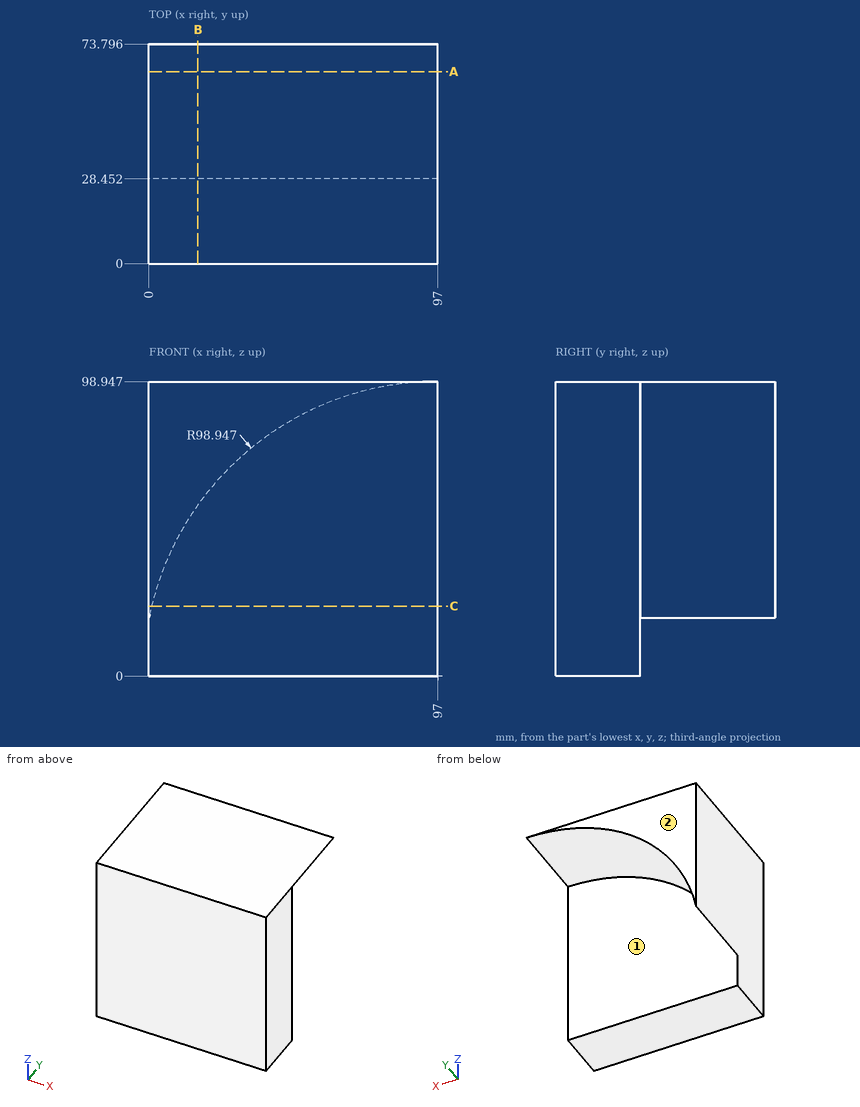
Source: three-view drawing plus pictorial views. Frame: mm from the lowest corner of the part. A direction names the side the tool comes from. Round coordinates to 2 decimals unless told otherwise and drop trailing zeros. Loops run counter-clockwise (first coordinate to the right, second up) from the corner with the lowest first, then second, coordinate; pieces in that order, holes last. Notation, with made-up numbers: M 47.25,45.25 L 100.25,45.25 A15 cw 100.25,52.25 Z; hole C 61.5,51 d8. An arc over 180 degrees is marked long. Answer as CSV lines item,"result". Start each with the question number.
(1) First-contact query: pin 1 (2 mm diameter, centred on x = 49, z = 72.5, fed in from +Y); pin 2 (12 mm diameter, centred on x = 26.5, y = 36, fed in from -Z) (1 decimal); pin 3 (1 mm diameter, centred on x = 51, y = 60.5, fed in from -Z). Flat tips, straight axial feed; report the tip coordinate or a pass-through.
(2) Reachability of the marked faces 1 and 2 from +Z, -Z, +X, -X, +Y, -Y: full face, straight path, thin tool, end or side. Return the list, or none.
(3) Section C-C, the plane z = 23.5. Output: boundary loops of the cut face in (x, y).
(4) Line query: line 1 (Y direction, x = 52.5, z = 86); line 2 (Z direction, x = 53, y = 58) (1 decimal); line 3 (Z direction, x = 9, y = 53). Output: solid intervals per line, ascending. Write a range as [from, to].
(5) Section A-A, the plane y = 64.5. Output: boundary loops of the cut face in (x, z), plus the area to 3 significant figures.
(6) Section B-B, the plane x = 16.5. Output: boundary loops of the cut face in (y, z).
Values found:
1,pin 1,"stops at y = 28.45"
1,pin 2,"stops at z = 62.8"
1,pin 3,"stops at z = 87.34"
2,face 1,"-Z, +X, +Y"
2,face 2,"+Z, -Z, +X, -X, +Y"
3,outline,"M 0,0 L 97,0 L 97,28.45 L 0.88,28.45 L 0.88,73.8 L 0,73.8 Z"
4,line 1,"y = [0, 28.45]"
4,line 2,"z = [88.6, 98.9]"
4,line 3,"z = [45.24, 98.95]"
5,outline,"M 0,19.53 A98.95 cw 97,98.95 L 0,98.95 Z"
5,area,"1,930 mm²"
6,outline,"M 0,0 L 28.45,0 L 28.45,57.53 L 73.8,57.53 L 73.8,98.95 L 0,98.95 Z"
